Build history of the part. All positions in model axes, mm. Face numbers are marked on the shaded views. Coordinates: 2 decimals unless noted, no trailing zeros. Loops run counter-clockwise (first coordinate to the right, second up) from the corner with the lowest first, then second, coordinate; pieces in that order, holes last. Notation, with made-up numbers: (6.25, -33) - (15.25, -33) arc R32 ccw to (15.25, -7) - close; hole circle Ø8 at (-24.75, 88). An arc over 180 degrees is marked (long way). One line per item, written item: value.
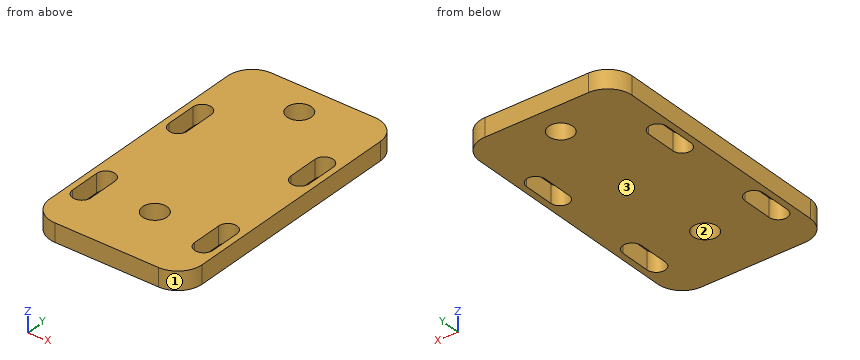
```python
from build123d import *

# Parameters (mm, degrees)
F1_DEPTH = 3
F2_R     = 2
F3_DEPTH = 3


with BuildPart() as f1:
    # F0 (on Top) → F1 (new body)
    with BuildSketch(Plane.XY):
        with BuildLine():
            Line((-8.5, -22.5), (8.5, -22.5))
            ThreePointArc((8.5, -22.5), (11.328427, -21.328427), (12.5, -18.5))
            Line((12.5, -18.5), (12.5, 18.5))
            ThreePointArc((12.5, 18.5), (11.328427, 21.328427), (8.5, 22.5))
            Line((8.5, 22.5), (-8.5, 22.5))
            ThreePointArc((-8.5, 22.5), (-11.328427, 21.328427), (-12.5, 18.5))
            Line((-12.5, 18.5), (-12.5, -18.5))
            ThreePointArc((-12.5, -18.5), (-11.328427, -21.328427), (-8.5, -22.5))
        make_face()
    extrude(amount=F1_DEPTH)

    # F2 (on face) → F3 (cut, through all)
    with BuildSketch(Plane.XY.offset(3)):
        with Locations((0, -12.5)):
            Circle(F2_R)
        with Locations((0, 17.5)):
            Circle(F2_R)
        with BuildLine():
            ThreePointArc((-8.5, 10), (-10, 11.5), (-11.5, 10))
            Line((-11.5, 10), (-11.5, 5))
            ThreePointArc((-11.5, 5), (-10, 3.5), (-8.5, 5))
            Line((-8.5, 5), (-8.5, 10))
        make_face()
        with BuildLine():
            ThreePointArc((11.5, 10), (10, 11.5), (8.5, 10))
            Line((8.5, 10), (8.5, 5))
            ThreePointArc((8.5, 5), (10, 3.5), (11.5, 5))
            Line((11.5, 5), (11.5, 10))
        make_face()
        with BuildLine():
            ThreePointArc((11.5, -10), (10, -8.5), (8.5, -10))
            Line((8.5, -10), (8.5, -15))
            ThreePointArc((8.5, -15), (10, -16.5), (11.5, -15))
            Line((11.5, -15), (11.5, -10))
        make_face()
        with BuildLine():
            ThreePointArc((-8.5, -10), (-10, -8.5), (-11.5, -10))
            Line((-11.5, -10), (-11.5, -15))
            ThreePointArc((-11.5, -15), (-10, -16.5), (-8.5, -15))
            Line((-8.5, -15), (-8.5, -10))
        make_face()
    extrude(amount=-F3_DEPTH, mode=Mode.SUBTRACT)


solid = f1.part
```
Item 1: Cut at A-A, the plane z = 1.9. Write the cut outline in (x, y), then the cut area to 3 significant figures.
Check result:
outline: (-12.5, -18.5) arc R4 ccw to (-8.5, -22.5) - (8.5, -22.5) arc R4 ccw to (12.5, -18.5) - (12.5, 18.5) arc R4 ccw to (8.5, 22.5) - (-8.5, 22.5) arc R4 ccw to (-12.5, 18.5) - close; hole (-11.5, -15) arc R1.5 ccw to (-8.5, -15) - (-8.5, -10) arc R1.5 ccw to (-11.5, -10) - close; hole (-11.5, 5) arc R1.5 ccw to (-8.5, 5) - (-8.5, 10) arc R1.5 ccw to (-11.5, 10) - close; hole circle Ø4 at (0, -12.5); hole circle Ø4 at (0, 17.5); hole (8.5, -15) arc R1.5 ccw to (11.5, -15) - (11.5, -10) arc R1.5 ccw to (8.5, -10) - close; hole (8.5, 5) arc R1.5 ccw to (11.5, 5) - (11.5, 10) arc R1.5 ccw to (8.5, 10) - close
area: 998 mm^2
Item 2: Pull direction Y, two halves, no side cores. Call the marked faces 1, 2 and 3: released by +Y, released by -Y, zero draft, split by the parting line, or undercut.
Check result:
face 1: released by -Y
face 2: undercut
face 3: zero draft
Item 3: Probe probe 1 along Y at (x, z) = (0, 1.35); probe 2 along Y at (x, z) = (0.5, 0.5); probe 3 along X at (y, z) = (-13.5, 1.45). List the from-to ranges inside material, lowest first. Write a range as from..to.
Check result:
probe 1: y = -22.5..-14.5, -10.5..15.5, 19.5..22.5
probe 2: y = -22.5..-14.44, -10.56..15.56, 19.44..22.5
probe 3: x = -12.5..-11.5, -8.5..-1.73, 1.73..8.5, 11.5..12.5
Item 4: Cut at D-D, the plane y = 11. Write the cut outline in (x, z), then the cut area to 3 significant figures.
Check result:
outline: (-12.5, 0) - (-11.12, 0) - (-11.12, 3) - (-12.5, 3) - close; (-8.88, 0) - (8.88, 0) - (8.88, 3) - (-8.88, 3) - close; (11.12, 0) - (12.5, 0) - (12.5, 3) - (11.12, 3) - close
area: 61.6 mm^2
Item 5: Cut at B-B, the plane y = -12.5. Write the cut outline in (x, z).
Check result:
outline: (-12.5, 0) - (-11.5, 0) - (-11.5, 3) - (-12.5, 3) - close; (-8.5, 0) - (-2, 0) - (-2, 3) - (-8.5, 3) - close; (2, 0) - (8.5, 0) - (8.5, 3) - (2, 3) - close; (11.5, 0) - (12.5, 0) - (12.5, 3) - (11.5, 3) - close
Item 6: Cut at C-C, the plane x = 0. Write the cut outline in (y, z).
Check result:
outline: (-22.5, 0) - (-14.5, 0) - (-14.5, 3) - (-22.5, 3) - close; (-10.5, 0) - (15.5, 0) - (15.5, 3) - (-10.5, 3) - close; (19.5, 0) - (22.5, 0) - (22.5, 3) - (19.5, 3) - close
